Check sheet for the modelled part. Datum: model origin and axes. Units: mm. A direction names the side the tool comes from. Round coordinates to 2 decimals unless told otherwise and drop trailing zeros. Write each loop counter-clockwise with the first axis right and the second up, starting at its lowest first coordinate (ties: lowest second). Pieces come first, ordered by that corner, then holes. Notation, with made-up numbers: (27, -25) - (68, -25) arc R16 ccw to (68, -1) - close; hole circle Ø6 at (89.25, 38.25). An arc over 180 degrees is marked (long way). Answer as a JSON object with one key per item and string values. Group by question number.
Item 1: Set-up check for faces 5 (the cylindrical face through (-75, 2, -28)), 6 (the flat face through (-25, 2, 25.5)): record each of +Z, -Z, +X, -X, +Y, -Y from which the full face is reachable in a straight line by a thin tool's end or side.
Item 2: Sectioned sample at B-B on x = -13. Record the boundary of the cut face in (y, z) (3 decimals), plus the area to 3 significant figures.
Item 3: Release check for a two-part mould opening along Z. For faces 1 (the cylindrical face through (9.5, 1.5, 22.9)), 2 (the flat face through (76, 1, 0)), 3 (the flat face through (0, 2, -25.5)), 4 (the cylindrical face through (-75, 2, 28)) record: pulls with the +Z half, pulls with the -Z half, needs draft (parallel to the pull), parting line crosses it, or undercut.
Item 4: Sectioned sample at A-A on x = 24.5. Record the boundary of the cut face in (y, z), plus the area to 3 significant figures.
Item 5: Thickness scan on line 1 (Z direction, x = -66, y = 2.2) (3 decimals); line 2 (Z direction, x = -1.5, y = 2.2); line 3 (X direction, y = 1.3, z = -9.5). Record the ranges inside material, lowest first.
Item 6: Sectioned sample at C-C on y = 0.6. Count the separate pieces of the cut face and the enclosed holes in it, plus the area to 3 significant figures.
```python
from build123d import *

# Parameters (mm, degrees)
SKETCH_1_W          = 152
SKETCH_1_H          = 60
EXTRUDE_1_DEPTH     = 3
CUT_EXTRUDE_1_REACH = 83.762
SKETCH_2_R          = 1.525
FILLET_1_R          = 5
CUT_EXTRUDE_2_REACH = 83.762
SKETCH_3_R          = 1.525
SKETCH_4_W          = 14
SKETCH_4_H          = 5
CUT_EXTRUDE_3_DEPTH = 3


with BuildPart() as part:
    # 草图1 → 凸台-拉伸1 (new body)
    with BuildSketch(Plane(origin=(0, 0, 0), x_dir=(1, 0, 0), z_dir=(0, 1, 0))):
        Rectangle(SKETCH_1_W, SKETCH_1_H)
    extrude(amount=EXTRUDE_1_DEPTH)

    # 草图2 → 切除-拉伸1 (cut, up to next)
    with BuildSketch(Plane(origin=(0, 3, 0), x_dir=(1, 0, 0), z_dir=(0, 1, 0)), mode=Mode.PRIVATE) as cut_extrude_1_sk1:
        with Locations(Location((-66, -24, 0), (0, 0, 270))):
            Circle(SKETCH_2_R)
    cut_extrude_1_tool1 = extrude(cut_extrude_1_sk1.sketch, amount=-CUT_EXTRUDE_1_REACH, mode=Mode.PRIVATE) & part.part
    # 草图2 → 切除-拉伸1 (cut, up to next)
    with BuildSketch(Plane(origin=(0, 3, 0), x_dir=(1, 0, 0), z_dir=(0, 1, 0)), mode=Mode.PRIVATE) as cut_extrude_1_sk2:
        with Locations(Location((-66, 24, 0), (0, 0, 270))):
            Circle(SKETCH_2_R)
    cut_extrude_1_tool2 = extrude(cut_extrude_1_sk2.sketch, amount=-CUT_EXTRUDE_1_REACH, mode=Mode.PRIVATE) & part.part
    # 草图2 → 切除-拉伸1 (cut, up to next)
    with BuildSketch(Plane(origin=(0, 3, 0), x_dir=(1, 0, 0), z_dir=(0, 1, 0)), mode=Mode.PRIVATE) as cut_extrude_1_sk3:
        with Locations(Location((66, -24, 0), (0, 0, 270))):
            Circle(SKETCH_2_R)
    cut_extrude_1_tool3 = extrude(cut_extrude_1_sk3.sketch, amount=-CUT_EXTRUDE_1_REACH, mode=Mode.PRIVATE) & part.part
    # 草图2 → 切除-拉伸1 (cut, up to next)
    with BuildSketch(Plane(origin=(0, 3, 0), x_dir=(1, 0, 0), z_dir=(0, 1, 0)), mode=Mode.PRIVATE) as cut_extrude_1_sk4:
        with Locations(Location((66, 24, 0), (0, 0, 270))):
            Circle(SKETCH_2_R)
    cut_extrude_1_tool4 = extrude(cut_extrude_1_sk4.sketch, amount=-CUT_EXTRUDE_1_REACH, mode=Mode.PRIVATE) & part.part
    add(cut_extrude_1_tool1.solids().sort_by_distance((-66, 3, 24))[0], mode=Mode.SUBTRACT)
    add(cut_extrude_1_tool2.solids().sort_by_distance((-66, 3, -24))[0], mode=Mode.SUBTRACT)
    add(cut_extrude_1_tool3.solids().sort_by_distance((66, 3, 24))[0], mode=Mode.SUBTRACT)
    add(cut_extrude_1_tool4.solids().sort_by_distance((66, 3, -24))[0], mode=Mode.SUBTRACT)

    # 圆角1
    fillet_1_edges = [part.edges().sort_by_distance(p)[0] for p in [
        (76, 1.5, 30),
        (-76, 1.5, 30),
        (-76, 1.5, -30),
        (76, 1.5, -30),
    ]]
    fillet(fillet_1_edges, radius=FILLET_1_R)

    # 草图3 → 切除-拉伸2 (cut, up to next)
    with BuildSketch(Plane(origin=(0, 3, 0), x_dir=(1, 0, 0), z_dir=(0, 1, 0)), mode=Mode.PRIVATE) as cut_extrude_2_sk1:
        with Locations(Location((-13, 10, 0), (0, 0, 270))):
            Circle(SKETCH_3_R)
    cut_extrude_2_tool1 = extrude(cut_extrude_2_sk1.sketch, amount=-CUT_EXTRUDE_2_REACH, mode=Mode.PRIVATE) & part.part
    # 草图3 → 切除-拉伸2 (cut, up to next)
    with BuildSketch(Plane(origin=(0, 3, 0), x_dir=(1, 0, 0), z_dir=(0, 1, 0)), mode=Mode.PRIVATE) as cut_extrude_2_sk2:
        with Locations(Location((-38, 15, 0), (0, 0, 270))):
            Circle(SKETCH_3_R)
    cut_extrude_2_tool2 = extrude(cut_extrude_2_sk2.sketch, amount=-CUT_EXTRUDE_2_REACH, mode=Mode.PRIVATE) & part.part
    # 草图3 → 切除-拉伸2 (cut, up to next)
    with BuildSketch(Plane(origin=(0, 3, 0), x_dir=(1, 0, 0), z_dir=(0, 1, 0)), mode=Mode.PRIVATE) as cut_extrude_2_sk3:
        with Locations(Location((-59, 17, 0), (0, 0, 270))):
            Circle(SKETCH_3_R)
    cut_extrude_2_tool3 = extrude(cut_extrude_2_sk3.sketch, amount=-CUT_EXTRUDE_2_REACH, mode=Mode.PRIVATE) & part.part
    # 草图3 → 切除-拉伸2 (cut, up to next)
    with BuildSketch(Plane(origin=(0, 3, 0), x_dir=(1, 0, 0), z_dir=(0, 1, 0)), mode=Mode.PRIVATE) as cut_extrude_2_sk4:
        with Locations(Location((-13, -10, 0), (0, 0, 270))):
            Circle(SKETCH_3_R)
    cut_extrude_2_tool4 = extrude(cut_extrude_2_sk4.sketch, amount=-CUT_EXTRUDE_2_REACH, mode=Mode.PRIVATE) & part.part
    # 草图3 → 切除-拉伸2 (cut, up to next)
    with BuildSketch(Plane(origin=(0, 3, 0), x_dir=(1, 0, 0), z_dir=(0, 1, 0)), mode=Mode.PRIVATE) as cut_extrude_2_sk5:
        with Locations(Location((-38, -15, 0), (0, 0, 270))):
            Circle(SKETCH_3_R)
    cut_extrude_2_tool5 = extrude(cut_extrude_2_sk5.sketch, amount=-CUT_EXTRUDE_2_REACH, mode=Mode.PRIVATE) & part.part
    # 草图3 → 切除-拉伸2 (cut, up to next)
    with BuildSketch(Plane(origin=(0, 3, 0), x_dir=(1, 0, 0), z_dir=(0, 1, 0)), mode=Mode.PRIVATE) as cut_extrude_2_sk6:
        with Locations(Location((-59, -17, 0), (0, 0, 270))):
            Circle(SKETCH_3_R)
    cut_extrude_2_tool6 = extrude(cut_extrude_2_sk6.sketch, amount=-CUT_EXTRUDE_2_REACH, mode=Mode.PRIVATE) & part.part
    # 草图3 → 切除-拉伸2 (cut, up to next)
    with BuildSketch(Plane(origin=(0, 3, 0), x_dir=(1, 0, 0), z_dir=(0, 1, 0)), mode=Mode.PRIVATE) as cut_extrude_2_sk7:
        with Locations(Location((13, -10, 0), (0, 0, 270))):
            Circle(SKETCH_3_R)
    cut_extrude_2_tool7 = extrude(cut_extrude_2_sk7.sketch, amount=-CUT_EXTRUDE_2_REACH, mode=Mode.PRIVATE) & part.part
    # 草图3 → 切除-拉伸2 (cut, up to next)
    with BuildSketch(Plane(origin=(0, 3, 0), x_dir=(1, 0, 0), z_dir=(0, 1, 0)), mode=Mode.PRIVATE) as cut_extrude_2_sk8:
        with Locations(Location((38, -15, 0), (0, 0, 270))):
            Circle(SKETCH_3_R)
    cut_extrude_2_tool8 = extrude(cut_extrude_2_sk8.sketch, amount=-CUT_EXTRUDE_2_REACH, mode=Mode.PRIVATE) & part.part
    # 草图3 → 切除-拉伸2 (cut, up to next)
    with BuildSketch(Plane(origin=(0, 3, 0), x_dir=(1, 0, 0), z_dir=(0, 1, 0)), mode=Mode.PRIVATE) as cut_extrude_2_sk9:
        with Locations(Location((59, -17, 0), (0, 0, 270))):
            Circle(SKETCH_3_R)
    cut_extrude_2_tool9 = extrude(cut_extrude_2_sk9.sketch, amount=-CUT_EXTRUDE_2_REACH, mode=Mode.PRIVATE) & part.part
    # 草图3 → 切除-拉伸2 (cut, up to next)
    with BuildSketch(Plane(origin=(0, 3, 0), x_dir=(1, 0, 0), z_dir=(0, 1, 0)), mode=Mode.PRIVATE) as cut_extrude_2_sk10:
        with Locations(Location((13, 10, 0), (0, 0, 270))):
            Circle(SKETCH_3_R)
    cut_extrude_2_tool10 = extrude(cut_extrude_2_sk10.sketch, amount=-CUT_EXTRUDE_2_REACH, mode=Mode.PRIVATE) & part.part
    # 草图3 → 切除-拉伸2 (cut, up to next)
    with BuildSketch(Plane(origin=(0, 3, 0), x_dir=(1, 0, 0), z_dir=(0, 1, 0)), mode=Mode.PRIVATE) as cut_extrude_2_sk11:
        with Locations(Location((38, 15, 0), (0, 0, 270))):
            Circle(SKETCH_3_R)
    cut_extrude_2_tool11 = extrude(cut_extrude_2_sk11.sketch, amount=-CUT_EXTRUDE_2_REACH, mode=Mode.PRIVATE) & part.part
    # 草图3 → 切除-拉伸2 (cut, up to next)
    with BuildSketch(Plane(origin=(0, 3, 0), x_dir=(1, 0, 0), z_dir=(0, 1, 0)), mode=Mode.PRIVATE) as cut_extrude_2_sk12:
        with Locations(Location((59, 17, 0), (0, 0, 270))):
            Circle(SKETCH_3_R)
    cut_extrude_2_tool12 = extrude(cut_extrude_2_sk12.sketch, amount=-CUT_EXTRUDE_2_REACH, mode=Mode.PRIVATE) & part.part
    add(cut_extrude_2_tool1.solids().sort_by_distance((-13, 3, -10))[0], mode=Mode.SUBTRACT)
    add(cut_extrude_2_tool2.solids().sort_by_distance((-38, 3, -15))[0], mode=Mode.SUBTRACT)
    add(cut_extrude_2_tool3.solids().sort_by_distance((-59, 3, -17))[0], mode=Mode.SUBTRACT)
    add(cut_extrude_2_tool4.solids().sort_by_distance((-13, 3, 10))[0], mode=Mode.SUBTRACT)
    add(cut_extrude_2_tool5.solids().sort_by_distance((-38, 3, 15))[0], mode=Mode.SUBTRACT)
    add(cut_extrude_2_tool6.solids().sort_by_distance((-59, 3, 17))[0], mode=Mode.SUBTRACT)
    add(cut_extrude_2_tool7.solids().sort_by_distance((13, 3, 10))[0], mode=Mode.SUBTRACT)
    add(cut_extrude_2_tool8.solids().sort_by_distance((38, 3, 15))[0], mode=Mode.SUBTRACT)
    add(cut_extrude_2_tool9.solids().sort_by_distance((59, 3, 17))[0], mode=Mode.SUBTRACT)
    add(cut_extrude_2_tool10.solids().sort_by_distance((13, 3, -10))[0], mode=Mode.SUBTRACT)
    add(cut_extrude_2_tool11.solids().sort_by_distance((38, 3, -15))[0], mode=Mode.SUBTRACT)
    add(cut_extrude_2_tool12.solids().sort_by_distance((59, 3, -17))[0], mode=Mode.SUBTRACT)

    # 草图4 → 切除-拉伸3 (cut)
    with BuildSketch(Plane(origin=(0, 3, 0), x_dir=(1, 0, 0), z_dir=(0, 1, 0))):
        with BuildLine():
            ThreePointArc((-57, -25.5), (-59.5, -23), (-57, -20.5))
            Line((-57, -20.5), (-57, -25.5))
        make_face()
        with Locations((-50, -23)):
            Rectangle(SKETCH_4_W, SKETCH_4_H)
        with BuildLine():
            ThreePointArc((-43, -20.5), (-40.5, -23), (-43, -25.5))
            Line((-43, -25.5), (-43, -20.5))
        make_face()
        with BuildLine():
            ThreePointArc((-32, -25.5), (-34.5, -23), (-32, -20.5))
            Line((-32, -20.5), (-32, -25.5))
        make_face()
        with Locations((-25, -23)):
            Rectangle(SKETCH_4_W, SKETCH_4_H)
        with BuildLine():
            ThreePointArc((-18, -20.5), (-15.5, -23), (-18, -25.5))
            Line((-18, -25.5), (-18, -20.5))
        make_face()
        with BuildLine():
            ThreePointArc((-7, -25.5), (-9.5, -23), (-7, -20.5))
            Line((-7, -20.5), (-7, -25.5))
        make_face()
        with Locations((0, -23)):
            Rectangle(SKETCH_4_W, SKETCH_4_H)
        with BuildLine():
            ThreePointArc((7, -20.5), (9.5, -23), (7, -25.5))
            Line((7, -25.5), (7, -20.5))
        make_face()
        with BuildLine():
            Line((18, -20.5), (18, -25.5))
            ThreePointArc((18, -25.5), (15.5, -23), (18, -20.5))
        make_face()
        with Locations((25, -23)):
            Rectangle(SKETCH_4_W, SKETCH_4_H)
        with BuildLine():
            Line((32, -20.5), (32, -25.5))
            ThreePointArc((32, -25.5), (34.5, -23), (32, -20.5))
        make_face()
        with BuildLine():
            Line((43, -20.5), (43, -25.5))
            ThreePointArc((43, -25.5), (40.5, -23), (43, -20.5))
        make_face()
        with Locations((50, -23)):
            Rectangle(SKETCH_4_W, SKETCH_4_H)
        with BuildLine():
            Line((57, -20.5), (57, -25.5))
            ThreePointArc((57, -25.5), (59.5, -23), (57, -20.5))
        make_face()
        with BuildLine():
            Line((-57, 20.5), (-57, 25.5))
            ThreePointArc((-57, 25.5), (-59.5, 23), (-57, 20.5))
        make_face()
        with Locations((-50, 23)):
            Rectangle(SKETCH_4_W, SKETCH_4_H)
        with BuildLine():
            Line((-43, 20.5), (-43, 25.5))
            ThreePointArc((-43, 25.5), (-40.5, 23), (-43, 20.5))
        make_face()
        with BuildLine():
            Line((-32, 20.5), (-32, 25.5))
            ThreePointArc((-32, 25.5), (-34.5, 23), (-32, 20.5))
        make_face()
        with Locations((-25, 23)):
            Rectangle(SKETCH_4_W, SKETCH_4_H)
        with BuildLine():
            Line((-18, 20.5), (-18, 25.5))
            ThreePointArc((-18, 25.5), (-15.5, 23), (-18, 20.5))
        make_face()
        with BuildLine():
            Line((-7, 20.5), (-7, 25.5))
            ThreePointArc((-7, 25.5), (-9.5, 23), (-7, 20.5))
        make_face()
        with Locations((0, 23)):
            Rectangle(SKETCH_4_W, SKETCH_4_H)
        with BuildLine():
            Line((7, 20.5), (7, 25.5))
            ThreePointArc((7, 25.5), (9.5, 23), (7, 20.5))
        make_face()
        with BuildLine():
            ThreePointArc((18, 20.5), (15.5, 23), (18, 25.5))
            Line((18, 25.5), (18, 20.5))
        make_face()
        with Locations((25, 23)):
            Rectangle(SKETCH_4_W, SKETCH_4_H)
        with BuildLine():
            ThreePointArc((32, 25.5), (34.5, 23), (32, 20.5))
            Line((32, 20.5), (32, 25.5))
        make_face()
        with BuildLine():
            ThreePointArc((43, 20.5), (40.5, 23), (43, 25.5))
            Line((43, 25.5), (43, 20.5))
        make_face()
        with Locations((50, 23)):
            Rectangle(SKETCH_4_W, SKETCH_4_H)
        with BuildLine():
            ThreePointArc((57, 25.5), (59.5, 23), (57, 20.5))
            Line((57, 20.5), (57, 25.5))
        make_face()
    extrude(amount=-CUT_EXTRUDE_3_DEPTH, mode=Mode.SUBTRACT)


solid = part.part
```
Completed:
{
 "1": {"face 5": "-Z, -X, +Y, -Y", "face 6": "+Y, -Y"},
 "2": {"outline": "(0, -30) - (3, -30) - (3, -11.525) - (0, -11.525) - close; (0, -8.475) - (3, -8.475) - (3, 8.475) - (0, 8.475) - close; (0, 11.525) - (3, 11.525) - (3, 30) - (0, 30) - close", "area": "162 mm²"},
 "3": {"face 1": "undercut", "face 2": "needs draft", "face 3": "undercut", "face 4": "pulls with the +Z half"},
 "4": {"outline": "(0, -30) - (3, -30) - (3, -25.5) - (0, -25.5) - close; (0, -20.5) - (3, -20.5) - (3, 20.5) - (0, 20.5) - close; (0, 25.5) - (3, 25.5) - (3, 30) - (0, 30) - close", "area": "150 mm²"},
 "5": {"line 1": "-30 to -25.525, -22.475 to 22.475, 25.525 to 30", "line 2": "-30 to -25.5, -20.5 to 20.5, 25.5 to 30", "line 3": "-76 to -14.44, -11.56 to 11.56, 14.44 to 76"},
 "6": {"separate pieces": "1", "enclosed holes": "26", "area": "8,090 mm²"}
}
